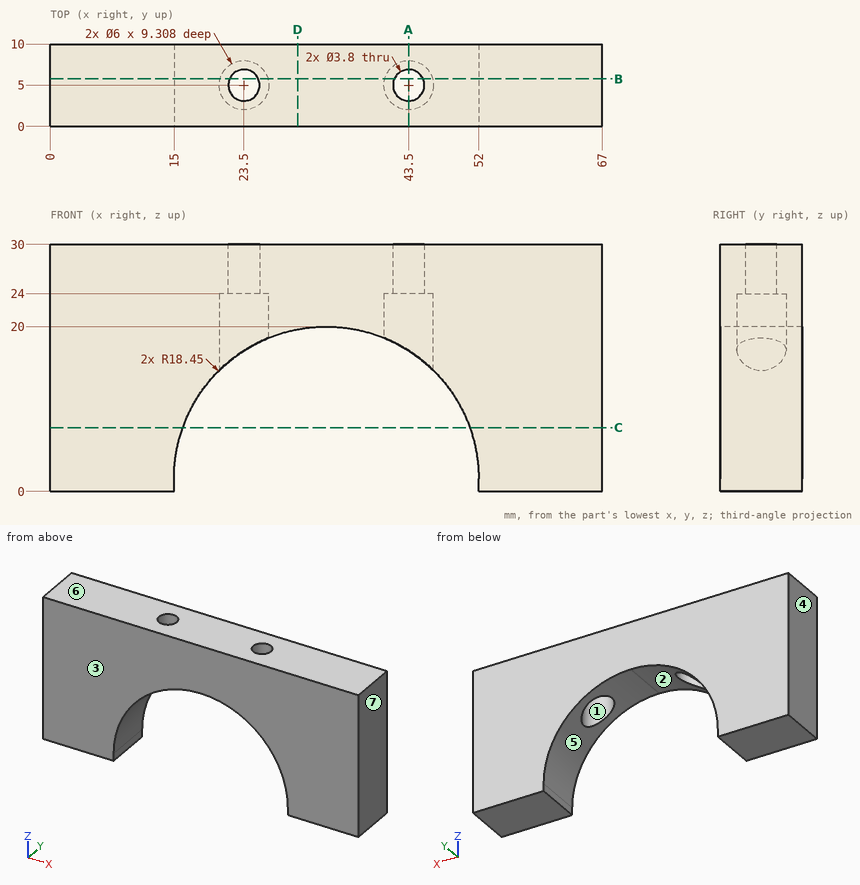
Geometry: see drawing. Coordinates: mm, zero at the bounding-box minimum. A direction names the side the tool comes from. Round coordinates to 2 decimals unless told otherwise and drop trailing zeros. Write each loop counter-clockwise with the first axis right and the second up, starting at its lowest first coordinate (ties: lowest second). Pieces come first, ordered by that corner, then holes.
1) Cut plane B-B (y = 5.75). Count the separate pieces of the cut face and the enclosed holes in it, then the cut area to 3 significant figures.
2) Contact query for flat-ended pins moving along their axis: P1, Ø5, axis at x = 34.5, y = 6, coming from the -Z side (1 decimal); P2, Ø3.5, axis at x = 43.5, y = 5, coming from the +Z side; P3, Ø5, axis at x = 23.5, y = 5, coming from the -Z side; P4, Ø1, axis at x = 36, y = 6, coming from the -Z side. Output: stop coordinate, or through.
3) Draft query along X for the marked faces 4, 5, 6 and 7. Return one class per face: pulls with the +X half, pulls with the -X half, needs draft (parallel to the pull), parting line crosses it, or undercut.
4) Reachability of the marked faces 1, 2 and 3 from +Z, -Z, +X, -X, +Y, -Y: full face, straight path, thin tool, end or side. Return the list, or none.
5) Cut plane C-C (z = 7.75). Return the cut outline in (x, y).
6) Cut plane D-D (x = 30). Return the cut outline in (y, z) (1 decimal), then the cut area to 3 significant figures.
7) Ray query, L1, parallel to X at y = 4, z = 2.25; L2, parallel to Y at x = 23.5, z = 26.85; L3, parallel to X at y = 2.75, z = 23 (1 decimal). Return the intervals inside material, ascending.
8) Cut plane A-A (x = 43.5). Return the cut outline in (y, z).
Geometry says:
1. separate pieces: 3
1. enclosed holes: 0
1. area: 1,290 mm2
2. P1: stops at z = 19.7
2. P2: passes through
2. P3: stops at z = 24
2. P4: stops at z = 19.76
3. face 4: pulls with the -X half
3. face 5: undercut
3. face 6: needs draft
3. face 7: pulls with the +X half
4. face 1: -Z
4. face 2: -Z, +Y, -Y
4. face 3: +Z, -Z, +X, -X, -Y
5. outline: (0, 0) - (16.07, 0) - (16.07, 10) - (0, 10) - close; (50.93, 0) - (67, 0) - (67, 10) - (50.93, 10) - close
6. outline: (0, 19.7) - (10, 19.7) - (10, 30) - (0, 30) - close
6. area: 103 mm2
7. L1: x = 0 to 15.01, 51.99 to 67
7. L2: y = 0 to 3.1, 6.9 to 10
7. L3: x = 0 to 21.5, 25.5 to 41.5, 45.5 to 67
8. outline: (0, 17.09) - (2, 17.09) - (2, 24) - (3.1, 24) - (3.1, 30) - (0, 30) - close; (6.9, 24) - (8, 24) - (8, 17.09) - (10, 17.09) - (10, 30) - (6.9, 30) - close
